The listing builds one solid part. Answer for the finished solid, in the listing's coordinates (mm). A direction names the side the tool comes from. Give positions to 0.01 mm unless a question says otherwise; leave off trailing zeros. Write each loop counter-clockwise with the first axis right and the second up, starting at its lowest first coordinate (ties: lowest second). Pieces come first, ordered by that corner, then holes. Notation, with made-up numbers: M 56.25,-8 L 97.25,-8 A20 ccw 97.25,19 Z; hole C -39,74.5 d8. An arc over 180 degrees is marked long. Return JSON: item names as keys, results as strings.
Autodesk Inventor part; units mm, degrees
ref_plane "YZ Plane" through (0, 0, 0) normal (1, 0, 0) x (0, 1, 0)
ref_plane "XZ Plane" through (0, 0, 0) normal (0, 1, 0) x (-1, 0, 0)
ref_plane "XY Plane" through (0, 0, 0) normal (0, 0, 1) x (1, 0, 0)
sketch "Sketch1" plane through (0, 0, 0) normal (1, 0, 0) x (0, 1, 0)
  circle A0 centre (0, 0) radius 16.5
  dimension "d0" = 33
extrude "Extrusion1" add sketch "Sketch1" along normal blind 22.7
sketch "Sketch2" plane through (22.7, 0, 0) normal (1, 0, 0) x (0, 0, -1)
  circle A0 centre (0, 0) radius 18.5
  dimension "d3" = 37
extrude "Extrusion2" add sketch "Sketch2" along normal blind 24
sketch "Sketch3" plane through (46.7, 0, 0) normal (1, 0, 0) x (0, 0, -1)
  circle A0 centre (0, 7) radius 7
  point P0 (0, 0)
  dimension "d6" = 14
  dimension "d7" = 7
extrude "Extrusion3" add sketch "Sketch3" along normal blind 6
sketch "Sketch4" plane through (52.7, 7, 0) normal (1, 0, 0) x (0, 0, -1)
  circle A0 centre (0, 0) radius 3
  point P0 (0, -7)
  dimension "d10" = 6
extrude "Extrusion4" add sketch "Sketch4" along normal blind 15.5
sketch "Sketch5" plane through (46.7, 0, 0) normal (1, 0, 0) x (0, 0, -1)
  circle A0 centre (-15.5, 0) radius 1.5
  circle A1 centre (0, 7) radius 7
  circle A2 centre (-7.75, -13.4234) radius 1.5
  circle A3 centre (7.75, -13.4234) radius 1.5
  circle A4 centre (15.5, 0) radius 1.5
  circle A5 centre (7.75, 13.4234) radius 1.5
  circle A6 centre (-7.75, 13.4234) radius 1.5
  point P0 (0, 0)
  dimension "d13" = 3
  dimension "d14" = 15.5
  dimension "d17" = 360
extrude "Extrusion5" cut sketch "Sketch5" against normal blind 10 contours A0 | A2 | A3 | A4 | A5 | A6
sketch "Sketch6" plane through (68.2, 7, 0) normal (1, 0, 0) x (0, 0, -1)
  line L0 (-3.2783, 3.4497) -> (2.5487, 3.4497)
  line L1 (2.5487, 3.4497) -> (2.5487, 1.5658)
  line L2 (2.5487, 1.5658) -> (-3.2783, 1.5658)
  line L3 (-3.2783, 1.5658) -> (-3.2783, 3.4497)
  point P0 (0, -7)
extrude "Extrusion6" cut sketch "Sketch6" against normal blind 10
properties part number "DCMotor"
Item 1: A cutting plane is placed at C-C, the plane x = 14. Write down the section's boundary in (y, z), plus the area to 3 significant figures.
Geometry results:
{"outline": "C 0,0 d33", "area": "855 mm2"}
Item 2: A cutting plane is placed at B-B, the plane y = -3. Write down the section's boundary in (x, z), plus the area to 3 significant figures.
Geometry results:
{"outline": "M 0,-16.22 L 22.7,-16.22 L 22.7,-18.26 L 46.7,-18.26 L 46.7,18.26 L 22.7,18.26 L 22.7,16.22 L 0,16.22 Z", "area": "1,610 mm2"}
Item 3: Which of the six approach directions +Z, -Z, +X, -X, +Y, -Y give full straight-line access (tool end or side, diameter ignored) to faces 1 (the cylindrical face through (42, 0, 17)), 2 (the flat face through (0, 0, 0)), 3 (the cylindrical face through (11.19, 15.24, 6.32))?
Geometry results:
{"face 1": "+X", "face 2": "+Z, -Z, -X, +Y, -Y", "face 3": "-X"}
Item 4: Determine the mould class of faces 4 (the cylindrical face through (49.658, 13.834, 1.517)), 5 (the cylindrical face through (41.77, -12.41, 8.856)), 6 (the flat face through (68.2, 6, 0)), 7 (the flat face through (36.7, 13, 8)) for opening direction Y: +Y half, -Y half, draft (parallel to the pull), parting line (faces both ways), or undercut.
Geometry results:
{"face 4": "parting line", "face 5": "undercut", "face 6": "draft", "face 7": "undercut"}
Item 5: Given pin 1 Ø3 at (y, z) = (0, 14) entering from +X; pin 2 Ø1 at (x, z) = (54.5, 1) entering from -Y; pin 3 Ø2.5 at (y, z) = (13.42, -7.75) entering from +X, each flat-ended and moving along its own axis, determine where each tip first touches the part or whether it passes through.
Geometry results:
{"pin 1": "stops at x = 46.7", "pin 2": "stops at y = 4.04", "pin 3": "stops at x = 36.7"}
Item 6: Find the intervals of material crossed by line 1 (Y direction, x = 43, z = 7.75); line 2 (X direction, y = -1, z = 7.5); line 3 (Z direction, x = 15.5, y = -7), in increasing order.
Geometry results:
{"line 1": "y = -16.8 to -14.92, -11.92 to 11.92, 14.92 to 16.8", "line 2": "x = 0 to 46.7", "line 3": "z = -14.94 to 14.94"}
Item 7: A cutting plane is placed at A-A, the plane z = 0. Write down the section's boundary in (x, y).
Geometry results:
{"outline": "M 0,-16.5 L 22.7,-16.5 L 22.7,-18.5 L 46.7,-18.5 L 46.7,0 L 52.7,0 L 52.7,4 L 68.2,4 L 68.2,8.57 L 58.2,8.57 L 58.2,10 L 52.7,10 L 52.7,14 L 46.7,14 L 46.7,18.5 L 22.7,18.5 L 22.7,16.5 L 0,16.5 Z"}
Item 8: A cutting plane is placed at D-D, the plane z = -15.5. Write down the section's boundary in (x, y), plus the area to 3 significant figures.
Geometry results:
{"outline": "M 0,-5.66 L 22.7,-5.66 L 22.7,-10.1 L 46.7,-10.1 L 46.7,-1.5 L 36.7,-1.5 L 36.7,1.5 L 46.7,1.5 L 46.7,10.1 L 22.7,10.1 L 22.7,5.66 L 0,5.66 Z", "area": "712 mm2"}
